The figure shows three views and two pictorial views of one solid part (mm, origin at its lowest corner). Answer the questions. A direction names the side the tool comes from. Give positions to 0.01 mm unless a question says otherwise; leave off trailing zeros. Loops run counter-clockwise (first coordinate to the right, second up) from the corner with the lowest first, then second, coordinate; pieces in that order, holes last. Notation, with made-up numbers: (53.5, -24) - (85.5, -24) arc R18 cw to (85.5, -19) - close; hole circle Ø5 at (-5.5, 49.25). An arc over 180 degrees is marked (long way). Use a Markdown table: item, result. Add a question column.
Item 1: For a pull along Z with two mould halves and no side action, classify the marked faces 1, 2 and 3 as +Z half, -Z half, draft (parallel to the pull), parting line (faces both ways), or undercut.
Item 2: Which of the six approach directions +Z, -Z, +X, -X, +Y, -Y give full straight-line access (tool end or side, diameter ignored) to the marked faces 4, 5 and 6?
Item 3: A cutting plane is placed at D-D (z = 29). Determine the outline of the cut face in (x, y), plus the area to 3 significant figures.
Item 4: Each of these flat-tipped pins is pushed along its axis until it touches: P1, Ø4, axis at y = 3.5, z = 55, coming from the -X side; P2, Ø6, axis at x = 51.5, y = 5, coming from the +Z side; P3, Ø1.5, axis at x = 7.5, z = 18.5, coming from the +Y side; P4, Ø2, axis at x = 12, z = 16, coming from the -Y side. Where does it stop, or does it pass through?
Item 5: Consider probe 1 along X at (y, z) = (14.5, 28); probe 2 along Y at (x, z) = (18, 35); probe 3 along Y at (x, z) = (4, 48.5). Determine where each line is inside the solid, lowest interval first. Write a range as [from, to].
Item 6: A cutting plane is placed at A-A (x = 35). Determine the outline of the cut face in (y, z).
Item 7: A cutting plane is placed at B-B (y = 8.5). Determine the outline of the cut face in (x, z), plus the area to 3 significant figures.
Item 8: A cutting plane is placed at C-C (y = 17.5). Determine the outline of the cut face in (x, z).
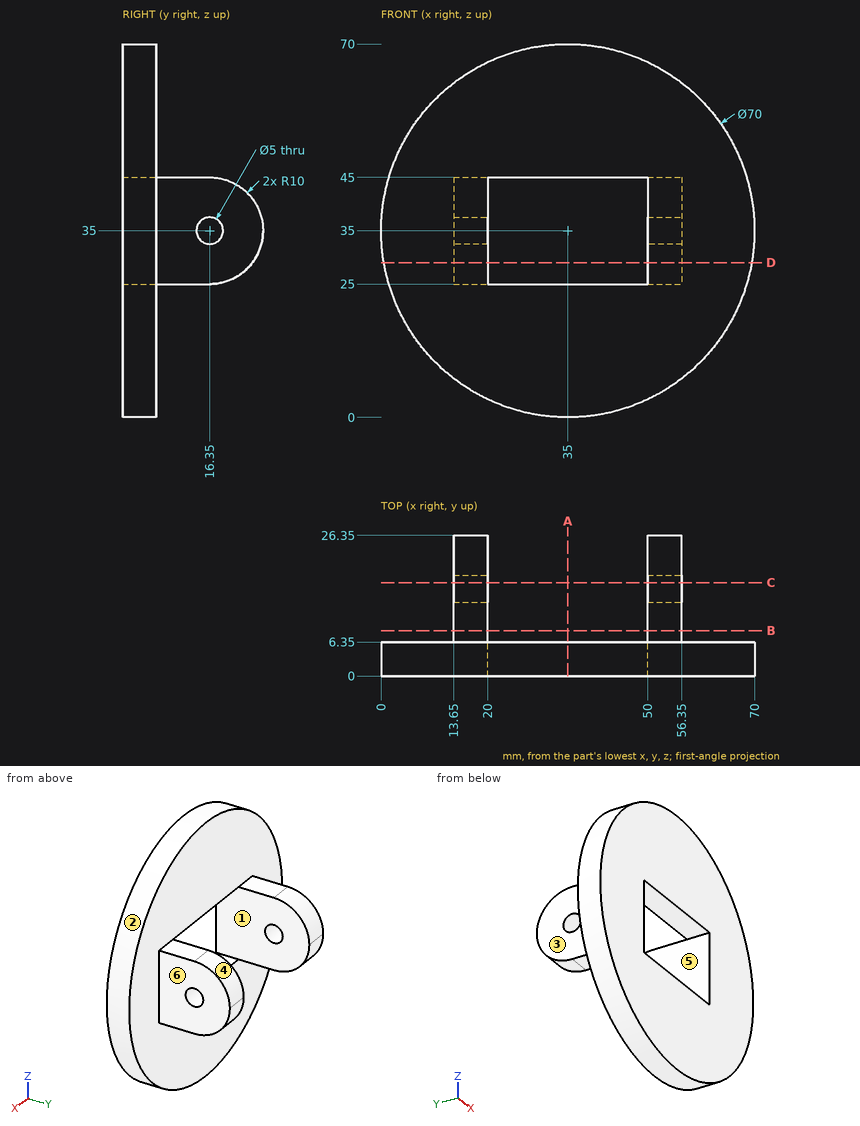
Geometry says:
| question | item | result |
|---|---|---|
| 1 | face 1 | undercut |
| 1 | face 2 | parting line |
| 1 | face 3 | draft |
| 2 | face 4 | +Z, +X, -X, +Y |
| 2 | face 5 | +Y, -Y |
| 2 | face 6 | +Z, -Z, +X, +Y |
| 3 | outline | (0.52, 0) - (20, 0) - (20, 24.35) - (13.65, 24.35) - (13.65, 6.35) - (0.52, 6.35) - close; (50, 0) - (69.48, 0) - (69.48, 6.35) - (56.35, 6.35) - (56.35, 24.35) - (50, 24.35) - close |
| 3 | area | 476 mm² |
| 4 | P1 | x = 4.98 |
| 4 | P2 | z = 67.29 |
| 4 | P3 | y = 6.35 |
| 4 | P4 | y = 0 |
| 5 | probe 1 | [13.65, 20], [50, 56.35] |
| 5 | probe 2 | [0, 13.85], [18.85, 26.35] |
| 5 | probe 3 | [0, 6.35] |
| 6 | outline | (0, 0) - (6.35, 0) - (6.35, 25) - (0, 25) - close; (0, 45) - (6.35, 45) - (6.35, 70) - (0, 70) - close |
| 7 | outline | (13.65, 25) - (20, 25) - (20, 45) - (13.65, 45) - close; (50, 25) - (56.35, 25) - (56.35, 45) - (50, 45) - close |
| 7 | area | 254 mm² |
| 8 | outline | (13.65, 25.07) - (20, 25.07) - (20, 32.78) - (13.65, 32.78) - close; (13.65, 37.22) - (20, 37.22) - (20, 44.93) - (13.65, 44.93) - close; (50, 25.07) - (56.35, 25.07) - (56.35, 32.78) - (50, 32.78) - close; (50, 37.22) - (56.35, 37.22) - (56.35, 44.93) - (50, 44.93) - close |
